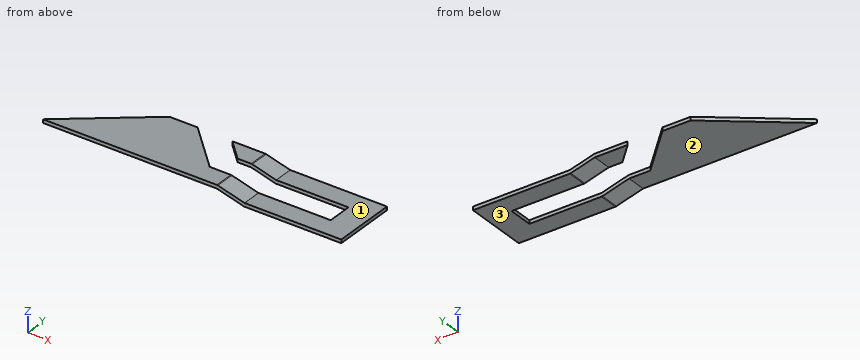
```python
from build123d import *

# Parameters (mm, degrees)
BASE_FLANGE1_DEPTH       = 5
EDGE_FLANGE1_DEPTH       = 27.5
EDGE_FLANGE2_DEPTH       = 27.5
EDGE_FLANGE2_START       = 62.5
EDGE_FLANGE2_2_OUTLINE_W = 137.70274344
EDGE_FLANGE2_2_OUTLINE_H = 5
EDGE_FLANGE2_2_DEPTH     = 27.5
EDGE_FLANGE2_START_2     = 27.5
EDGE_FLANGE2_3_OUTLINE_W = 35
EDGE_FLANGE2_3_OUTLINE_H = 5
EDGE_FLANGE2_3_DEPTH     = 35
EDGE_FLANGE3_DEPTH       = 27.5
EDGE_FLANGE4_DEPTH       = 27.5
EDGE_FLANGE4_START       = 5
EDGE_FLANGE4_FLAT_DEPTH  = 5


# Read off the part's stored shape, not the designer's step: Edge-Flange2
# Sheet-metal steps are written as plain solids
with BuildPart() as part:
    # Sketch1 → Base-Flange1 (new body)
    with BuildSketch(Plane.XY):
        Polygon((0, 0), (-117.7971995, 0), (-2.7971995, 90), (37.2028005, 90), (99.7028005, 27.5), (129.7028005, 27.5), (129.7028005, 0), align=None)
    extrude(amount=-BASE_FLANGE1_DEPTH)

    # Edge-Flange1 section (across the edge) → Edge-Flange1 (add)
    with BuildSketch(Plane(origin=(129.79977573, 27.5, -5), x_dir=(-0.2588190451025146, 0, -0.96592582628907), z_dir=(0, -1, 0))):
        with BuildLine():
            Line((-5, 0.09697523), (-5, 39.341737512))
            Line((-5, 39.341737512), (0, 39.341737512))
            Line((0, 39.341737512), (0, 0.09697523))
            ThreePointArc((0, 0.09697523), (0.006301715, 0.000829637), (0.025099036, -0.093670879))
            Line((0.025099036, -0.093670879), (-4.804530095, -1.387766104))
            ThreePointArc((-4.804530095, -1.387766104), (-4.950922592, -0.651801325), (-5, 0.09697523))
        make_face()
    extrude(amount=EDGE_FLANGE1_DEPTH)

    # Edge-Flange2 outline → Edge-Flange2 (add)
    with BuildSketch(Plane(origin=(0, 0, 0), x_dir=(1, 0, 0), z_dir=(0, 1, 0))):
        with BuildLine():
            ThreePointArc((169.285717378, 15.37786084), (168.536940824, 15.328783432), (167.800976044, 15.182390936))
            Line((167.800976044, 15.182390936), (169.09507127, 10.352761804))
            ThreePointArc((169.09507127, 10.352761804), (169.189571785, 10.371559125), (169.285717378, 10.37786084))
            Line((169.285717378, 10.37786084), (306.891485589, 10.37786084))
            Line((306.891485589, 10.37786084), (306.891485589, 15.37786084))
            Line((306.891485589, 15.37786084), (169.285717378, 15.37786084))
        make_face()
    extrude(amount=EDGE_FLANGE2_DEPTH)



with BuildPart() as body_2:
    # Edge-Flange2 2 outline → Edge-Flange2 2 (new body)
    with BuildSketch(Plane(origin=(0, 0, 0), x_dir=(1, 0, 0), z_dir=(0, 1, 0)).offset(EDGE_FLANGE2_START)):
        with Locations((238.040113869, 12.87786084)):
            Rectangle(EDGE_FLANGE2_2_OUTLINE_W, EDGE_FLANGE2_2_OUTLINE_H)
    extrude(amount=EDGE_FLANGE2_2_DEPTH)


with BuildPart() as part_1:
    add(part.part)

    add(body_2.part)  # Edge-Flange2 3 merges body 2
    # Edge-Flange2 3 outline → Edge-Flange2 3 (add)
    with BuildSketch(Plane(origin=(0, 0, 0), x_dir=(1, 0, 0), z_dir=(0, 1, 0)).offset(EDGE_FLANGE2_START_2)):
        with Locations((289.391485589, 12.87786084)):
            Rectangle(EDGE_FLANGE2_3_OUTLINE_W, EDGE_FLANGE2_3_OUTLINE_H)
    extrude(amount=EDGE_FLANGE2_3_DEPTH)

    # Edge-Flange3 section (across the edge) → Edge-Flange3 (add)
    with BuildSketch(Plane(origin=(169.091766919, 90, -10.37786084), x_dir=(0.2588190451025146, 0, 0.96592582628907), z_dir=(0, -1, 0))):
        with BuildLine():
            Line((-5, 0.09697523), (-5, 35.422092475))
            Line((-5, 35.422092475), (0, 35.422092475))
            Line((0, 35.422092475), (0, 0.09697523))
            ThreePointArc((0, 0.09697523), (0.006301715, 0.000829637), (0.025099036, -0.093670879))
            Line((0.025099036, -0.093670879), (-4.804530095, -1.387766104))
            ThreePointArc((-4.804530095, -1.387766104), (-4.950922592, -0.651801325), (-5, 0.09697523))
        make_face()
    extrude(amount=EDGE_FLANGE3_DEPTH)

    # Edge-Flange4 bend section (across the edge) → Edge-Flange4 (add)
    with BuildSketch(Plane(origin=(133.488886871, 62.5, -6.014478786), x_dir=(0, 0, -1), z_dir=(0, 1, 0))):
        with BuildLine():
            Line((-5, 0.09697523), (0, 0.09697523))
            ThreePointArc((0, 0.09697523), (0.006301715, 0.000829637), (0.025099036, -0.093670879))
            Line((0.025099036, -0.093670879), (-4.804530095, -1.387766104))
            ThreePointArc((-4.804530095, -1.387766104), (-4.950922592, -0.651801325), (-5, 0.09697523))
        make_face()
    extrude(amount=EDGE_FLANGE4_DEPTH)

    # Edge-Flange4 profile (on flange) → Edge-Flange4 flat (add)
    with BuildSketch(Plane(origin=(133.488886871, 0, -6.014478786), x_dir=(0, 1, 0), z_dir=(0, 0, 1)).offset(EDGE_FLANGE4_START)):
        Polygon((62.5, 19.382282567), (62.5, 0.09697523), (90, 0.09697523), (90, 46.882282567), align=None)
    extrude(amount=-EDGE_FLANGE4_FLAT_DEPTH)


solid = part_1.part
```
CAD build for the part. Positions are in the model's coordinates, mm. Face numbers are marked on the shaded views. A direction names the side the tool comes from. Coordinates: 2 decimals unless noted, no trailing zeros. Order: outer loops, then holes, each group sorted by start corner. A loop starts at its lowest first (then second) coordinate and runs counter-clockwise, first axis right, second up. Notation, with made-up numbers: (21, 6) -> (48, 6) arc R20 cw to (48, 45) -> close; hole circle Ø7 at (-38.5, 72). An arc over 180 degrees is marked (long way). Use one line per item in the form item = value. Start each with the question number.
1) Band-saw the part on A-A on y = 44. Give the cut face in (x, z), then the cut area to 3 significant figures.
2) Band-saw the part on D-D on x = 5. Give the cut face in (y, z), then the cut area to 3 significant figures.
3) Tool access for the marked faces 1, 2 and 3: list every direction of +Z, -Z, +X, -X, +Y, -Y with a clear straight run to the whole face (end or side of a thin tool).
4) Drop flat-ended pins along their axis: pin 1 (6 mm diameter, centred on x = 252, y = 72, fed in from +Z); pin 2 (8 mm diameter, centred on x = 121, y = 79, fed in from -Z); pin 3 (5.5 mm diameter, centred on y = 53, z = -12.5, fed in from -X). Give the stop position or say it passes through.
5) Drill centre lines: L1, parallel to Y at x = 260.5, z = -11.75; L2, parallel to X at y = 35.5, z = -10.75; L3, parallel to Z at x = 73.5, y = 48.5. Where is each one in solid material? Low to high. Write a range as [from, to].
6) Band-saw the part on B-B on x = 159. Give the cut face in (y, z), then the cut area to 3 significant figures.
7) Band-saw the part on C-C on y = 73.5. Give the cut face in (x, z).
Entries:
q1.outline = (-61.57, -5) -> (83.2, -5) -> (83.2, 0) -> (-61.57, 0) -> close; (271.89, -15.38) -> (306.89, -15.38) -> (306.89, -10.38) -> (271.89, -10.38) -> close
q1.area = 899 mm2
q2.outline = (0, -5) -> (90, -5) -> (90, 0) -> (0, 0) -> close
q2.area = 450 mm2
q3.face_1 = +Z, +X, +Y, -Y
q3.face_2 = -Z, -X, -Y
q3.face_3 = -Z, +X, -X, +Y, -Y
q4.pin_1 = -10.38
q4.pin_2 = -6.01
q4.pin_3 = 271.89
q5.L1 = [0, 27.5], [62.5, 90]
q5.L2 = [271.89, 306.89]
q5.L3 = [-5, 0]
q6.outline = (0, -12.82) -> (27.5, -12.82) -> (27.5, -7.65) -> (0, -7.65) -> close; (62.5, -12.85) -> (90, -12.85) -> (90, -7.67) -> (62.5, -7.67) -> close
q6.area = 285 mm2
q7.outline = (-23.88, -5) -> (53.7, -5) -> (53.7, 0) -> (-23.88, 0) -> close; (103.11, -6.01) -> (133.39, -6.01) arc R0.74 cw to (133.58, -6.04) -> (167.7, -15.18) arc R5.74 ccw to (169.19, -15.38) -> (306.89, -15.38) -> (306.89, -10.38) -> (169.19, -10.38) arc R0.74 cw to (169, -10.35) -> (134.88, -1.21) arc R5.74 ccw to (133.39, -1.01) -> (103.11, -1.01) -> close
